Source: CAD feature listing. Evaluate the final solid. Frame: model axes, mm. Give positions to 0.01 mm unless a question says otherwise; leave off trailing zeros. Loops run counter-clockwise (first coordinate to the right, second up) from the corner with the lowest first, then second, coordinate; pieces in that order, holes last. Notation, with made-up numbers: (74, 76) -> (113, 76) arc R20 cw to (113, 101) -> close; hole circle Ø4 at (-35, -8.5). An arc over 180 degrees is marked (long way). Return JSON: item names as keys, results as strings. Group by question number.
```python
from build123d import *

# Parameters (mm, degrees)
SKETCH1_R           = 0.5
BOSS_EXTRUDE1_DEPTH = 10


with BuildPart() as part:
    # Sketch1 → Boss-Extrude1 (new body)
    with BuildSketch(Plane(origin=(0, 0, 0), x_dir=(1, 0, 0), z_dir=(0, 1, 0))):
        Circle(SKETCH1_R)
    extrude(amount=BOSS_EXTRUDE1_DEPTH)

    # Sketch2 → Cut-Revolve2 (revolve, cut)
    with BuildSketch(Plane.XY):
        with BuildLine():
            Line((0.5, 9.866025404), (0.5, 10.1))
            Line((0.5, 10.1), (0, 10.1))
            Line((0, 10.1), (0, 10))
            ThreePointArc((0, 10), (0.258819045, 9.965925826), (0.5, 9.866025404))
        make_face()
        with BuildLine():
            Line((0.5, -0.1), (0, -0.1))
            Line((0, -0.1), (0, 0))
            ThreePointArc((0, 0), (0.258819045, 0.034074174), (0.5, 0.133974596))
            Line((0.5, 0.133974596), (0.5, -0.1))
        make_face()
    revolve(axis=Axis((0, 0, 0), (0, 1, 0)), mode=Mode.SUBTRACT)

    # Sketch3 → Cut-Revolve3 (revolve, cut)
    with BuildSketch(Plane.XY):
        with BuildLine():
            Line((-0.5, 9.5), (-0.41266406, 9.910883293))
            ThreePointArc((-0.41266406, 9.910883293), (-0.456882894, 9.889526852), (-0.5, 9.866025404))
            Line((-0.5, 9.866025404), (-0.5, 9.5))
        make_face()
        with BuildLine():
            Line((-0.5, 0.133974596), (-0.5, 0.5))
            Line((-0.5, 0.5), (-0.41266406, 0.089116707))
            ThreePointArc((-0.41266406, 0.089116707), (-0.456882894, 0.110473148), (-0.5, 0.133974596))
        make_face()
    revolve(axis=Axis((0, 0, 0), (0, 1, 0)), mode=Mode.SUBTRACT)


solid = part.part
```
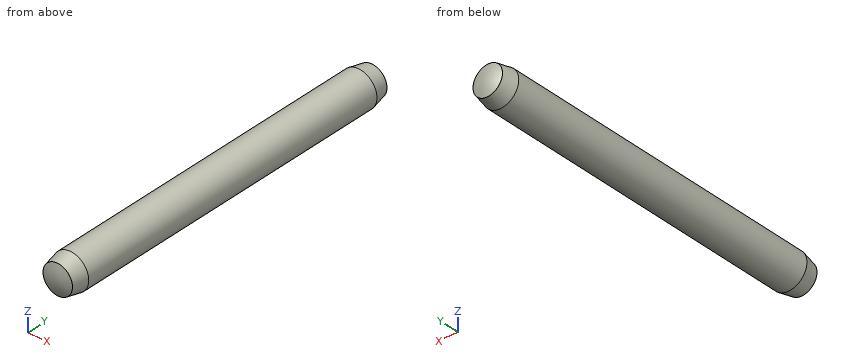
1) Cut plane A-A on x = 0. Return loops of the section in (y, z), then the cut area to 3 significant figures.
2) Cut plane B-B on z = 0. Return loops of the section in (x, y), then the cut area to 3 significant figures.
3) Cut plane C-C on y = 7.75. Return loops of the section in (x, z), then the cut area to 3 significant figures.
4) Material intervals for line 1 (Y direction, x = 0, z = -0.05); line 2 (X direction, y = 9, z = -0.05); line 3 (X direction, y = 3.75, z = 0.4), sorted ascending.
Calculated:
{
 "1": {"outline": "(0.09, -0.41) -> (0.5, -0.5) -> (9.5, -0.5) -> (9.91, -0.41) arc R1 ccw to (9.91, 0.41) -> (9.5, 0.5) -> (0.5, 0.5) -> (0.09, 0.41) arc R1 ccw to start", "area": "9.85 mm2"},
 "2": {"outline": "(-0.5, 0.5) -> (-0.41, 0.09) arc R1 ccw to (0.41, 0.09) -> (0.5, 0.5) -> (0.5, 9.5) -> (0.41, 9.91) arc R1 ccw to (-0.41, 9.91) -> (-0.5, 9.5) -> close", "area": "9.85 mm2"},
 "3": {"outline": "circle Ø1 at (0, 0)", "area": "0.785 mm2"},
 "4": {"line 1": "0 to 10", "line 2": "-0.5 to 0.5", "line 3": "-0.3 to 0.3"}
}
